from build123d import *

# Parameters (mm, degrees)
SKETCH_W          = 10
SKETCH_H          = 29.8
PAD_DEPTH         = 10
COPYSKETCH001_R   = 2
COPYSKETCH001_R_2 = 15
POCKET_DEPTH      = 10.001
FILLET_R          = 15
SKETCH001_R       = 1.5
POCKET001_DEPTH   = 10.001


with BuildPart() as part:
    # Sketch → Pad (new body)
    with BuildSketch(Plane.XZ):
        Polygon((0, 0), (0, 57.4), (10, 57.4), (10, 87.2), (0, 87.2), (0, 117.2), (10, 117.2), (10, 147), (0, 147), (0, 177), (10, 177), (10, 200), (170, 200), (170, 177), (180, 177), (180, 200), (410, 200), (410, 177), (420, 177), (420, 147), (410, 147), (410, 117.2), (420, 117.2), (420, 87.2), (410, 87.2), (410, 57.4), (420, 57.4), (420, 0), align=None)
        with Locations((175, 132.1)):
            Rectangle(SKETCH_W, SKETCH_H, mode=Mode.SUBTRACT)
        with Locations((175, 72.3)):
            Rectangle(SKETCH_W, SKETCH_H, mode=Mode.SUBTRACT)
    extrude(amount=PAD_DEPTH)

    # CopySketch001 → Pocket (cut, through all)
    with BuildSketch(Plane.XZ):
        with Locations((73, 163.6)):
            Circle(COPYSKETCH001_R)
        with Locations((107, 163.6)):
            Circle(COPYSKETCH001_R)
        with Locations((107, 136.4)):
            Circle(COPYSKETCH001_R)
        with Locations((73, 136.4)):
            Circle(COPYSKETCH001_R)
        with Locations((90, 150)):
            Circle(COPYSKETCH001_R_2)
    extrude(amount=POCKET_DEPTH, mode=Mode.SUBTRACT)

    # Fillet
    fillet_edges = [part.edges().sort_by_distance(p)[0] for p in [
        (0, -5, 0),
    ]]
    fillet(fillet_edges, radius=FILLET_R)

    # Sketch001 → Pocket001 (cut, through all)
    with BuildSketch(Plane.XZ):
        with Locations((199, 175.5)):
            Circle(SKETCH001_R)
        with Locations((356, 175.5)):
            Circle(SKETCH001_R)
        with Locations((356, 60.5)):
            Circle(SKETCH001_R)
        with Locations((199, 60.5)):
            Circle(SKETCH001_R)
        Polygon((195, 170), (360, 170), (360, 69), (352, 69), (352, 64), (332, 64), (332, 69), (297, 69), (297, 67), (257, 67), (257, 69), (195, 69), align=None)
    extrude(amount=POCKET001_DEPTH, mode=Mode.SUBTRACT)


solid = part.part
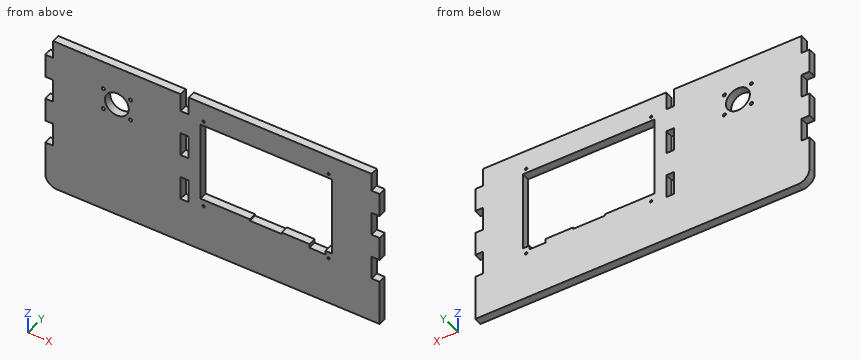
Source: CAD feature listing. Evaluate the final solid. Frame: model axes, mm. Round coordinates to 2 decimals unless told otherwise and drop trailing zeros. Loops run counter-clockwise (first coordinate to the right, second up) from the corner with the lowest first, then second, coordinate; pieces in that order, holes last.
Q1. Ray query, line 1 (Z direction, x = 199, y = -9.5); line 2 (X direction, y = -6.75, z = 175.5); line 3 (Z direction, x = 107, y = -4.25). Return the intervals inside material, ascending.
Q2. Section A-A, the plane x = 293. Return loops of the section in (y, z), plus the area to 3 significant figures.
Q3. Section D-D, the plane y = -6.75. State how many separate pieces and enclosed holes the cut face has, plus the area to 3 significant figures.
Q4. Section B-B, the plane z = 184.5. Return loops of the section in (x, y).
Q5. Section C-C, the plane z = 127.5. Return loops of the section in (x, y).
Q6. First-contact query: P1, Ø5.5, axis at y = -3.5, z = 66, coming from the +X side; P2, Ø4, axis at y = -7.5, z = 130, coming from the -X side; P3, Ø5, axis at x = 176.5, y = -6, coming from the +Z side; P4, Ø4, axis at x = 376, z = 141, coming from the +Y side. Flat tips, straight axial feed; report the tip coordinate or a pass-through.
Solutions:
1. line 1: z = 0 to 59, 62 to 69, 170 to 174, 177 to 200
1. line 2: x = 0 to 197.5, 200.5 to 354.5, 357.5 to 420
1. line 3: z = 0 to 134.4, 138.4 to 161.6, 165.6 to 200
2. outline: (-10, 0) - (0, 0) - (0, 67) - (-10, 67) - close; (-10, 170) - (0, 170) - (0, 200) - (-10, 200) - close
2. area: 970 mm2
3. separate pieces: 1
3. enclosed holes: 12
3. area: 63,800 mm2
4. outline: (10, -10) - (170, -10) - (170, 0) - (10, 0) - close; (180, -10) - (410, -10) - (410, 0) - (180, 0) - close
5. outline: (10, -10) - (170, -10) - (170, 0) - (10, 0) - close; (180, -10) - (195, -10) - (195, 0) - (180, 0) - close; (360, -10) - (410, -10) - (410, 0) - (360, 0) - close
6. P1: stops at x = 410
6. P2: stops at x = 10
6. P3: stops at z = 177
6. P4: stops at y = 0
